Verification items for the finished model (mm, model axes). A direction names the side the tool comes from. Round coordinates to 2 decimals unless told otherwise and drop trailing zeros. Order: outer loops, then holes, each group sorted by start corner. A loop starts at its lowest first (then second) coordinate and runs counter-clockwise, first axis right, second up. Notation, with made-up numbers: (13, 68.5) -> (69, 68.5) arc R22 cw to (69, 86.5) -> close; hole circle Ø3 at (-4, 3.5). An arc over 180 degrees is marked (long way). Put each result on its own line as item: value.
from build123d import *

# Parameters (mm, degrees)
ESBO_O1_W                = 32
ESBO_O1_H                = 5
ESBO_O1_R                = 1.5
RESSALTO_EXTRUS_O1_DEPTH = 4
ESBO_O3_W                = 4
ESBO_O3_H                = 5
RESSALTO_EXTRUS_O2_DEPTH = 44
PADR_O_LINEAR1_COUNT     = 2
PADR_O_LINEAR1_PITCH     = 40
ESBO_O4_R                = 1.285304246
CORTE_EXTRUS_O1_DEPTH    = 39


with BuildPart() as part:
    # Esboço1 → Ressalto-extrusão1 (new body)
    with BuildSketch(Plane.XY):
        Rectangle(ESBO_O1_W, ESBO_O1_H)
        with Locations((-10, 0)):
            Circle(ESBO_O1_R, mode=Mode.SUBTRACT)
        with BuildLine():
            ThreePointArc((5, 1.118033989), (2.5, 0), (5, -1.118033989))
            ThreePointArc((5, -1.118033989), (6, -1.5), (7, -1.118033989))
            ThreePointArc((7, -1.118033989), (8, -1.5), (9, -1.118033989))
            ThreePointArc((9, -1.118033989), (11.5, 0), (9, 1.118033989))
            ThreePointArc((9, 1.118033989), (8, 1.5), (7, 1.118033989))
            ThreePointArc((7, 1.118033989), (6, 1.5), (5, 1.118033989))
        make_face(mode=Mode.SUBTRACT)
    ressalto_extrus_o1 = extrude(amount=RESSALTO_EXTRUS_O1_DEPTH)

    # Esboço3 → Ressalto-extrusão2 (add)
    with BuildSketch(Plane.XY.offset(4)):
        with Locations((18, 0)):
            Rectangle(ESBO_O3_W, ESBO_O3_H)
    ressalto_extrus_o2 = extrude(amount=-RESSALTO_EXTRUS_O2_DEPTH)

    # Padrão linear1: Ressalto-extrusão1 ×2
    with Locations(*[(0, 0, -i * PADR_O_LINEAR1_PITCH) for i in range(1, PADR_O_LINEAR1_COUNT)]):
        add(ressalto_extrus_o1)

    # Espelhar1: Ressalto-extrusão2 across plane
    add(ressalto_extrus_o2.mirror(Plane(origin=(0, 0, 0), x_dir=(0, 0, 1), z_dir=(1, 0, 0))))

    # Esboço4 → Corte-extrusão1 (cut)
    with BuildSketch(Plane(origin=(20, 0, 0), x_dir=(0, 0, -1), z_dir=(1, 0, 0))):
        with Locations((8.412908062, 0)):
            Circle(ESBO_O4_R)
        with Locations((25.412908062, 0)):
            Circle(ESBO_O4_R)
    extrude(amount=-CORTE_EXTRUS_O1_DEPTH, mode=Mode.SUBTRACT)


solid = part.part
Item 1: Section check A-A on x = -14. Record the boundary of the cut face in (y, z).
Check sheet entries:
outline: (-2.5, -40) -> (2.5, -40) -> (2.5, -36) -> (-2.5, -36) -> close; (-2.5, 0) -> (2.5, 0) -> (2.5, 4) -> (-2.5, 4) -> close
Item 2: Section check D-D on z = -8.5. Record the boundary of the cut face in (x, y).
Check sheet entries:
outline: (-20, -2.5) -> (-16, -2.5) -> (-16, -1.28) -> (-19, -1.28) -> (-19, 1.28) -> (-16, 1.28) -> (-16, 2.5) -> (-20, 2.5) -> close; (16, -2.5) -> (20, -2.5) -> (20, -1.28) -> (16, -1.28) -> close; (16, 1.28) -> (20, 1.28) -> (20, 2.5) -> (16, 2.5) -> close
Item 3: Gauge pin test, flat ends, axial feed: pin 1 Ø0.8 at (y, z) = (0, -25) entering from +X; pin 2 Ø1.5 at (y, z) = (0, -9.5) entering from +X. Record the tip position at first contact, or that the pin passes through.
Check sheet entries:
pin 1: stops at x = -19
pin 2: stops at x = 20
Item 4: Section check C-C on z = -1. Record the boundary of the cut face in (x, y).
Check sheet entries:
outline: (-20, -2.5) -> (-16, -2.5) -> (-16, 2.5) -> (-20, 2.5) -> close; (16, -2.5) -> (20, -2.5) -> (20, 2.5) -> (16, 2.5) -> close
Item 5: Tool access check on faces 1 (the cylindrical face through (6, -1.5, 2)), 2 (the flat face through (-19, 0, -8)), 3 (the flat face through (16, 0, -18)). Record the directions out of +Z, -Z, +X, -X, +Y, -Y that give a thin tool (end or side, any length) a straight path to the whole face; none if there is none.
Check sheet entries:
face 1: +Z, -Z
face 2: +X
face 3: +Y, -Y
Item 6: Material ranges on L1, parallel to X at y = -1.3, z = -28.5; L2, parallel to Y at x = -10, z = 1; L3, parallel to Z at x = 3, y = 1.25, recorded low to high. Write a range as [from, to].
Check sheet entries:
L1: x = [-20, -16], [16, 20]
L2: y = [-2.5, -1.5], [1.5, 2.5]
L3: z = [-40, -36], [0, 4]
Item 7: Release check for a two-part mould opening along Y. For faces 4 (the flat face through (18, -2.5, -18)), 5 (the cylindrical face through (6, 1.5, 2)), 6 (the cylindrical face through (8, -1.5, 2)), 7 (the flat face through (0, 0, 0)) record: +Y half, -Y half, draft (parallel to the pull), parting line (faces both ways), or undercut.
Check sheet entries:
face 4: -Y half
face 5: undercut
face 6: undercut
face 7: draft
Item 8: Section check B-B on x = 10. Record the boundary of the cut face in (y, z), then the cut area to 3 significant figures.
Check sheet entries:
outline: (-2.5, -40) -> (-1.5, -40) -> (-1.5, -36) -> (-2.5, -36) -> close; (-2.5, 0) -> (-1.5, 0) -> (-1.5, 4) -> (-2.5, 4) -> close; (1.5, -40) -> (2.5, -40) -> (2.5, -36) -> (1.5, -36) -> close; (1.5, 0) -> (2.5, 0) -> (2.5, 4) -> (1.5, 4) -> close
area: 16.0 mm^2
